Could you check a few things on this model? Use its own coordinates, in mm. A direction names the side the tool comes from. Give positions to 0.01 mm unless a question says otherwise; leave off trailing zeros. Write each loop counter-clockwise with the first axis right and the second up, starting at its lowest first coordinate (ties: lowest second). Pieces come first, ordered by that corner, then holes. Notation, with made-up numbers: M -23,70 L 23,70 A29 cw 23,102 Z; hole C -12,67.25 d2. An arc over 180 degrees is marked long. Use one line per item in the form item = value.
from build123d import *

# Parameters (mm, degrees)
SKETCH1_W           = 20
SKETCH1_H           = 47
BOSS_EXTRUDE3_DEPTH = 5
SKETCH2_W           = 10.1
SKETCH2_H           = 47.2
SKETCH2_W_2         = 50.2
SKETCH2_H_2         = 5
CUT_EXTRUDE1_DEPTH  = 15
SKETCH3_R           = 2.55
CUT_EXTRUDE3_DEPTH  = 10
SKETCH4_W           = 5
SKETCH4_H           = 28.5
BOSS_EXTRUDE4_DEPTH = 34
CUT_EXTRUDE4_DEPTH  = 130.812364588
FILLET1_R           = 5
SKETCH6_W           = 5.5
SKETCH6_H           = 28.5
BOSS_EXTRUDE5_DEPTH = 5
SKETCH9_R           = 2.5
CUT_EXTRUDE7_DEPTH  = 180
CHAMFER1_SIZE       = 25
SKETCH10_W          = 10
SKETCH10_H          = 10
SKETCH10_W_2        = 12
SKETCH10_H_2        = 12
CUT_EXTRUDE8_DEPTH  = 106.906798649


with BuildPart() as part:
    # Sketch1 → Boss-Extrude3 (new body)
    with BuildSketch(Plane(origin=(0, 0, 0), x_dir=(1, 0, 0), z_dir=(0, 1, 0))):
        Polygon((55, 50), (-55, 50), (-55, 21.75), (-55, -21.75), (-55, -80), (-20, -80), (2.5, -80), (20, -80), (42.5, -80), (55, -80), (55, -21.75), (55, 21.75), align=None)
        Rectangle(SKETCH1_W, SKETCH1_H, mode=Mode.SUBTRACT)
    extrude(amount=BOSS_EXTRUDE3_DEPTH)

    # Sketch2 → Cut-Extrude1 (cut)
    with BuildSketch(Plane.XZ):
        with Locations((-20.05, 0)):
            Rectangle(SKETCH2_W, SKETCH2_H)
        with Locations((20.05, 0)):
            Rectangle(SKETCH2_W, SKETCH2_H)
        with Locations((0, 36)):
            Rectangle(SKETCH2_W_2, SKETCH2_H_2)
    extrude(amount=-CUT_EXTRUDE1_DEPTH, mode=Mode.SUBTRACT)

    # Sketch3 → Cut-Extrude3 (cut)
    with BuildSketch(Plane(origin=(0, 5, 0), x_dir=(1, 0, 0), z_dir=(0, 1, 0))):
        with Locations(Location((-45, 25, 0), (0, 0, 270))):
            Circle(SKETCH3_R)
        with Locations(Location((-45, -60, 0), (0, 0, 270))):
            Circle(SKETCH3_R)
        with Locations(Location((45, -60, 0), (0, 0, 270))):
            Circle(SKETCH3_R)
        with Locations(Location((45, 25, 0), (0, 0, 270))):
            Circle(SKETCH3_R)
    extrude(amount=-CUT_EXTRUDE3_DEPTH, mode=Mode.SUBTRACT)

    # Sketch4 → Boss-Extrude4 (add)
    with BuildSketch(Plane(origin=(0, 5, 0), x_dir=(1, 0, 0), z_dir=(0, 1, 0))):
        with Locations((-37, -10)):
            Rectangle(SKETCH4_W, SKETCH4_H)
        with Locations((37, -10)):
            Rectangle(SKETCH4_W, SKETCH4_H)
    extrude(amount=BOSS_EXTRUDE4_DEPTH)

    # Sketch5 → Cut-Extrude4 (cut, through all)
    with BuildSketch(Plane.ZY.offset(39.5)):
        with BuildLine():
            ThreePointArc((4.7, 15), (4.202081528, 16.202081528), (3, 16.7))
            Line((3, 16.7), (3, 15))
            Line((3, 15), (4.7, 15))
        make_face()
        with BuildLine():
            Line((3, 15), (3, 16.7))
            ThreePointArc((3, 16.7), (1.797918472, 13.797918472), (4.7, 15))
            Line((4.7, 15), (3, 15))
        make_face()
        with BuildLine():
            Line((3, 27.3), (3, 29))
            Line((3, 29), (4.7, 29))
            ThreePointArc((4.7, 29), (1.797918472, 30.202081528), (3, 27.3))
        make_face()
        with BuildLine():
            Line((4.7, 29), (3, 29))
            Line((3, 29), (3, 27.3))
            ThreePointArc((3, 27.3), (4.202081528, 27.797918472), (4.7, 29))
        make_face()
        with BuildLine():
            ThreePointArc((18.7, 29), (17, 30.7), (15.3, 29))
            Line((15.3, 29), (17, 29))
            Line((17, 29), (17, 27.3))
            ThreePointArc((17, 27.3), (18.202081528, 27.797918472), (18.7, 29))
        make_face()
        with BuildLine():
            Line((17, 29), (15.3, 29))
            ThreePointArc((15.3, 29), (15.797918472, 27.797918472), (17, 27.3))
            Line((17, 27.3), (17, 29))
        make_face()
        with BuildLine():
            ThreePointArc((18.7, 15), (18.202081528, 16.202081528), (17, 16.7))
            Line((17, 16.7), (17, 15))
            Line((17, 15), (15.3, 15))
            ThreePointArc((15.3, 15), (17, 13.3), (18.7, 15))
        make_face()
        with BuildLine():
            Line((17, 15), (17, 16.7))
            ThreePointArc((17, 16.7), (15.797918472, 16.202081528), (15.3, 15))
            Line((15.3, 15), (17, 15))
        make_face()
    extrude(amount=-CUT_EXTRUDE4_DEPTH, mode=Mode.SUBTRACT)

    # Fillet1
    fillet1_edges = [part.edges().sort_by_distance(p)[0] for p in [
        (-34.5, 5, 10),
        (34.5, 5, 10),
    ]]
    fillet(fillet1_edges, radius=FILLET1_R)

    # Sketch6 → Boss-Extrude5 (add)
    with BuildSketch(Plane(origin=(0, 5, 0), x_dir=(1, 0, 0), z_dir=(0, 1, 0))):
        with Locations((-57.75, -10)):
            Rectangle(SKETCH6_W, SKETCH6_H)
        with Locations((57.75, -10)):
            Rectangle(SKETCH6_W, SKETCH6_H)
    extrude(amount=-BOSS_EXTRUDE5_DEPTH)

    # Sketch9 → Cut-Extrude7 (cut)
    with BuildSketch(Plane(origin=(0, 5, 0), x_dir=(1, 0, 0), z_dir=(0, 1, 0))):
        with Locations(Location((-45, 40, 0), (0, 0, 270))):
            Circle(SKETCH9_R)
        with Locations(Location((45, 40, 0), (0, 0, 270))):
            Circle(SKETCH9_R)
        with Locations(Location((-25, 40, 0), (0, 0, 270))):
            Circle(SKETCH9_R)
        with Locations(Location((25, 40, 0), (0, 0, 270))):
            Circle(SKETCH9_R)
    extrude(amount=-CUT_EXTRUDE7_DEPTH, mode=Mode.SUBTRACT)

    # Chamfer1
    chamfer1_edges = [part.edges().sort_by_distance(p)[0] for p in [
        (55, 2.5, 80),
        (-55, 2.5, 80),
    ]]
    chamfer(chamfer1_edges, length=CHAMFER1_SIZE)

    # Sketch10 → Cut-Extrude8 (cut, through all)
    with BuildSketch(Plane(origin=(0, 5, 0), x_dir=(1, 0, 0), z_dir=(0, 1, 0))):
        with Locations((0, 33.5)):
            Rectangle(SKETCH10_W, SKETCH10_H)
        with Locations((-19.1, -56.5)):
            Rectangle(SKETCH10_W_2, SKETCH10_H_2)
        with Locations((19.1, -56.5)):
            Rectangle(SKETCH10_W_2, SKETCH10_H_2)
    extrude(amount=-CUT_EXTRUDE8_DEPTH, mode=Mode.SUBTRACT)


solid = part.part
1) I want a section at B-B, the plane x = 45. Please give me the cut outline in (y, z).
Checked values:
outline = M 0,-50 L 5,-50 L 5,-42.5 L 0,-42.5 Z; M 0,-37.5 L 5,-37.5 L 5,-27.55 L 0,-27.55 Z; M 0,-22.45 L 5,-22.45 L 5,57.45 L 0,57.45 Z; M 0,62.55 L 5,62.55 L 5,65 L 0,65 Z
2) I want a section at C-C, the plane z = -14. Please give me the cut outline in (x, y), plus the area to 3 significant figures.
Checked values:
outline = M -55,0 L -25.1,0 L -25.1,5 L -55,5 Z; M -15,0 L -10,0 L -10,5 L -15,5 Z; M 10,0 L 15,0 L 15,5 L 10,5 Z; M 25.1,0 L 55,0 L 55,5 L 25.1,5 Z
area = 349 mm2
3) Thinking about a two-plate mould opening in Z: for faces 6 (the flat face through (34.5, 24, 10)), 7 (the flat face through (-13.1, 3, 57)), 8 (the flat face through (-58, 3, -4.25)), which applies, released by +Z, released by -Z, zero draft, split by the parting line, or undercut?
Checked values:
face_6 = zero draft
face_7 = undercut
face_8 = released by -Z
4) For faces 1 (the flat face through (39.5, 22, 10)), 2 (the flat face through (-37, 22, -4.25)), 3 (the flat face through (60.5, 3, 10)), 4 (the flat face through (58, 3, 24.25)), 5 (the flat face through (19, 3, 62.5)), which set-ups out of +Z, -Z, +X, -X, +Y, -Y let a thin tool reach every point of the face, with its end or its side?
Checked values:
face_1 = +Z, -Z, +X, +Y
face_2 = -Z, +X, -X, +Y
face_3 = +Z, -Z, +X, +Y, -Y
face_4 = +Z, +X, +Y, -Y
face_5 = +Y, -Y
5) If I drill on L1, parallel to Y at x = -37.75, z = 3; L2, parallel to X at y = 1, z = -25; L3, parallel to X at y = 2.2, z = -40, over which ranges is the centre line in solid material (lowest first)?
Checked values:
L1 = 0 to 13.3, 16.7 to 27.3, 30.7 to 39
L2 = -55 to -47.55, -42.45 to 42.45, 47.55 to 55
L3 = -55 to -47.5, -42.5 to -27.5, -22.5 to 22.5, 27.5 to 42.5, 47.5 to 55
6) I want a section at A-A, the plane z = 60. Please give me the cut outline in (x, y).
Checked values:
outline = M -50,0 L -47.55,0 L -47.55,5 L -50,5 Z; M -42.45,0 L -25.1,0 L -25.1,5 L -42.45,5 Z; M -13.1,0 L 13.1,0 L 13.1,5 L -13.1,5 Z; M 25.1,0 L 42.45,0 L 42.45,5 L 25.1,5 Z; M 47.55,0 L 50,0 L 50,5 L 47.55,5 Z
7) I want a section at D-D, the plane y = 19.5. Please give me the cut outline in (x, z).
Checked values:
outline = M -39.5,-4.25 L -34.5,-4.25 L -34.5,24.25 L -39.5,24.25 Z; M 34.5,-4.25 L 39.5,-4.25 L 39.5,24.25 L 34.5,24.25 Z
8) For pin 1 Ø10 at (y, z) = (9.5, 56.5) entering from +X; pin 2 Ø4 at (y, z) = (1.5, 44.5) entering from -X; pin 3 Ø4 at (y, z) = (3.5, 57.5) entering from -X, each with a flat end and sliding along its axis, tell me the tip position at first contact or that it passes through.
Checked values:
pin_1 = 55
pin_2 = -55
pin_3 = -54.5
